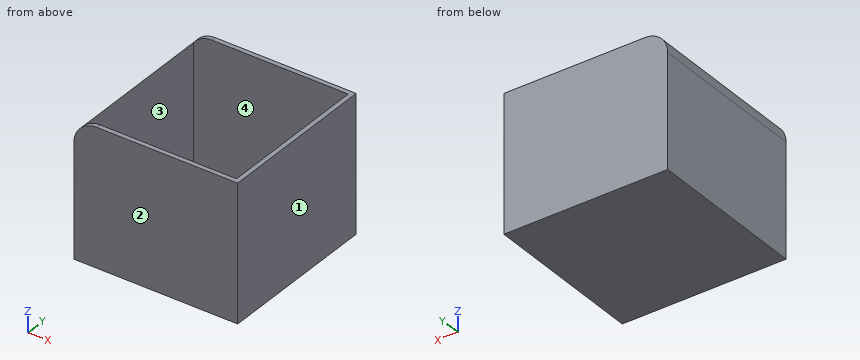
```python
from build123d import *

# Parameters (mm, degrees)
F0_W        = 72
F0_H        = 72
F1_DEPTH    = 60
F2_W        = 68
F2_H        = 68
F3_DEPTH    = 58
F4_T1_DEPTH = 122.8


# Not quite as in the source:
# - a fillet or chamfer that OpenCascade refuses, or shapes differently, is made with other operations: its cross-section is extruded or revolved along the edge and cut away or added


with BuildPart() as f1:
    # F0 (on Top) → F1 (new body)
    with BuildSketch(Plane.XY):
        with Locations((24.6826619834, 21.6548714693)):
            Rectangle(F0_W, F0_H)
    extrude(amount=F1_DEPTH)

    # F2 (on face) → F3 (cut)
    with BuildSketch(Plane.XY.offset(60)):
        with Locations((24.6826619834, 21.6548714693)):
            Rectangle(F2_W, F2_H)
    extrude(amount=-F3_DEPTH, mode=Mode.SUBTRACT)

    # F4: fillet of radius 10.16 on 1 edges, made by hand

    # F4_s2 → F4_t1 (cut)
    with BuildSketch(Plane.XZ.offset(-83.0548714693)):
        with BuildLine():
            ThreePointArc((-1.1573380166, 60), (-8.3415429135, 57.0242048969), (-11.3173380166, 49.84))
            Line((-11.3173380166, 49.84), (-11.3173380166, 60))
            Line((-11.3173380166, 60), (-1.1573380166, 60))
        make_face()
    extrude(amount=F4_T1_DEPTH, mode=Mode.SUBTRACT)


solid = f1.part
```
Part model, mm, in its own coordinate system. Face numbers are marked on the shaded views. Give positions to 0.01 mm unless a question says otherwise; leave off trailing zeros. Order: outer loops, then holes, each group sorted by start corner. A loop starts at its lowest first (then second) coordinate and runs counter-clockwise, first axis right, second up. Notation, with made-up numbers: M 29,-2 L 79,-2 A18 ccw 79,26 Z; hole C 32,10.5 d8. An arc over 180 degrees is marked long. Use a Markdown table: item, result. Add a question column.
(1) Drop flat-ended pins along their axis: P1, Ø6, axis at x = 46, y = 39, coming from the -Z side; P2, Ø10, axis at x = 28.5, y = 34.5, coming from the +Z side. Give the stop position or say it passes through.
(2) Probe line 1 along Y through (x, z) = (25.5, 10); line 2 along X through (y, z) = (24, 15); line 3 along Z through (x, y) = (57, 5.5). List the from-to ranges inside material, lowest first. Write a range as [from, to].
(3) Saw through at B-B, the plane y = 17.5. Give the cut face in (x, z), and give its area (3 significant figures).
(4) Saw through at A-A, the plane z = 29. Give the cut face in (x, y).
(5) Saw through at C-C, the plane x = -4. Give the cut face in (y, z).
(6) Mould opens along X. For the marked faces 1, 2, 3 and 4 say: +X half, -X half, draft (parallel to the pull), parting line (faces both ways), or undercut.
Answer key:
| question | item | result |
|---|---|---|
| 1 | P1 | z = 0 |
| 1 | P2 | z = 2 |
| 2 | line 1 | [-14.35, -12.35], [55.65, 57.65] |
| 2 | line 2 | [-11.32, -9.32], [58.68, 60.68] |
| 2 | line 3 | [0, 2] |
| 3 | outline | M -11.32,0 L 60.68,0 L 60.68,60 L 58.68,60 L 58.68,2 L -9.32,2 L -9.32,55.89 A10.16 ccw -11.32,49.84 Z |
| 3 | area | 364 mm^2 |
| 4 | outline | M -11.32,-14.35 L 60.68,-14.35 L 60.68,57.65 L -11.32,57.65 Z; hole M -9.32,-12.35 L 58.68,-12.35 L 58.68,55.65 L -9.32,55.65 Z |
| 5 | outline | M -14.35,0 L 57.65,0 L 57.65,59.59 L 55.65,59.59 L 55.65,2 L -12.35,2 L -12.35,59.59 L -14.35,59.59 Z |
| 6 | face 1 | +X half |
| 6 | face 2 | draft |
| 6 | face 3 | undercut |
| 6 | face 4 | undercut |
